```python
from build123d import *

# Parameters (mm, degrees)
SKETCH_1_R          = 27
SKETCH_1_R_2        = 1.5
EXTRUDE_1_DEPTH     = 1
FILLET_1_R          = 3
SKETCH_2_R          = 1.55
CUT_EXTRUDE_1_DEPTH = 3


with BuildPart() as part:
    # 草图1 → 凸台-拉伸1 (new body, symmetric)
    with BuildSketch(Plane.XY):
        Circle(SKETCH_1_R)
        with Locations((-12.63922466, 15.5)):
            Circle(SKETCH_1_R_2, mode=Mode.SUBTRACT)
        with Locations((12.63922466, 15.5)):
            Circle(SKETCH_1_R_2, mode=Mode.SUBTRACT)
        with Locations((-12.63922466, -15.5)):
            Circle(SKETCH_1_R_2, mode=Mode.SUBTRACT)
        with Locations((12.63922466, -15.5)):
            Circle(SKETCH_1_R_2, mode=Mode.SUBTRACT)
        with BuildLine():
            Line((-20.174241002, 13), (-9.327379053, 13))
            ThreePointArc((-9.327379053, 13), (0, 16), (9.327379053, 13))
            Line((9.327379053, 13), (20.174241002, 13))
            ThreePointArc((20.174241002, 13), (24, 0), (20.174241002, -13))
            Line((20.174241002, -13), (9.327379053, -13))
            ThreePointArc((9.327379053, -13), (0, -16), (-9.327379053, -13))
            Line((-9.327379053, -13), (-20.174241002, -13))
            ThreePointArc((-20.174241002, -13), (-24, 0), (-20.174241002, 13))
        make_face(mode=Mode.SUBTRACT)
    extrude(amount=EXTRUDE_1_DEPTH, both=True)

    # 圆角1
    fillet_1_edges = [part.edges().sort_by_distance(p)[0] for p in [
        (-20.174241002, 13, 0),
        (-20.174241002, -13, 0),
        (-9.327379053, -13, 0),
        (9.327379053, -13, 0),
        (20.174241002, -13, 0),
        (20.174241002, 13, 0),
        (9.327379053, 13, 0),
        (-9.327379053, 13, 0),
    ]]
    fillet(fillet_1_edges, radius=FILLET_1_R)

    # 草图2 → 切除-拉伸1 (cut, through all)
    with BuildSketch(Plane.XY.offset(1)):
        with Locations((-5, 19.5)):
            Circle(SKETCH_2_R)
        with Locations((5, 19.5)):
            Circle(SKETCH_2_R)
        with Locations((-5, -19.5)):
            Circle(SKETCH_2_R)
        with Locations((5, -19.5)):
            Circle(SKETCH_2_R)
    extrude(amount=-CUT_EXTRUDE_1_DEPTH, mode=Mode.SUBTRACT)


solid = part.part
```
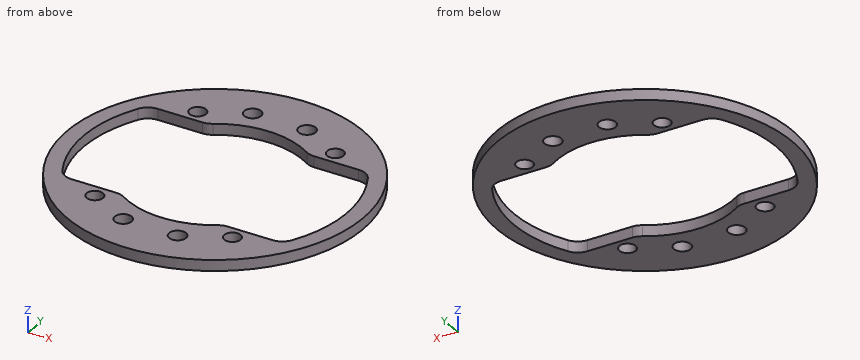
Here's how the part is built. I have some questions about the finished solid (model axes, mm). Give positions to 0.01 mm unless a question says otherwise; leave off trailing zeros. Loops run counter-clockwise (first coordinate to the right, second up) from the corner with the lowest first, then second, coordinate; pieces in that order, holes last. Notation, with made-up numbers: (-3, 22.5) -> (18, 22.5) arc R26 cw to (18, 40.5) -> close; hole circle Ø1 at (-2.75, -14.5). An arc over 180 degrees is marked (long way). Use one line per item in the form item = value. Start each with the question number.
1) Imagine slicing it at B-B (y = 0). Please give me the cut outline in (x, z).
2) Imagine slicing it at D-D (y = 19.5). Please give me the cut outline in (x, z), then the cut area to 3 significant figures.
3) Imagine slicing it at C-C (x = 0). Please give me the cut outline in (y, z).
4) For P1, Ø0.6, axis at x = 13, z = 0.5, coming from the +Y side; P2, Ø2.5, axis at x = -5, y = 19.5, coming from the +Z side, each with a flat end and sliding along its axis, tell me the tip position at first contact or that it passes through.
5) Imagine slicing it at A-A (z = -0.65). Count the separate pieces of the cut face and the enclosed holes in it, then the cut area to 3 significant figures.
6) Please list where these lines run through material, in increasing order: line 1 along Y through (x, z) = (-13, 0.85); line 2 along Y through (x, z) = (-5, -0.35); line 3 along Y through (x, z) = (7.5, 0.05).
Check values:
q1.outline = (-27, -1) -> (-24, -1) -> (-24, 1) -> (-27, 1) -> close; (24, -1) -> (27, -1) -> (27, 1) -> (24, 1) -> close
q2.outline = (-18.67, -1) -> (-6.55, -1) -> (-6.55, 1) -> (-18.67, 1) -> close; (-3.45, -1) -> (3.45, -1) -> (3.45, 1) -> (-3.45, 1) -> close; (6.55, -1) -> (18.67, -1) -> (18.67, 1) -> (6.55, 1) -> close
q2.area = 62.3 mm^2
q3.outline = (-27, -1) -> (-16, -1) -> (-16, 1) -> (-27, 1) -> close; (16, -1) -> (27, -1) -> (27, 1) -> (16, 1) -> close
q4.P1 = 23.83
q4.P2 = through
q5.separate_pieces = 1
q5.enclosed_holes = 9
q5.area = 973 mm^2
q6.line_1 = -23.66 to -16.96, -14.04 to -13, 13 to 14.04, 16.96 to 23.66
q6.line_2 = -26.53 to -21.05, -17.95 to -15.2, 15.2 to 17.95, 21.05 to 26.53
q6.line_3 = -25.94 to -14.13, 14.13 to 25.94
